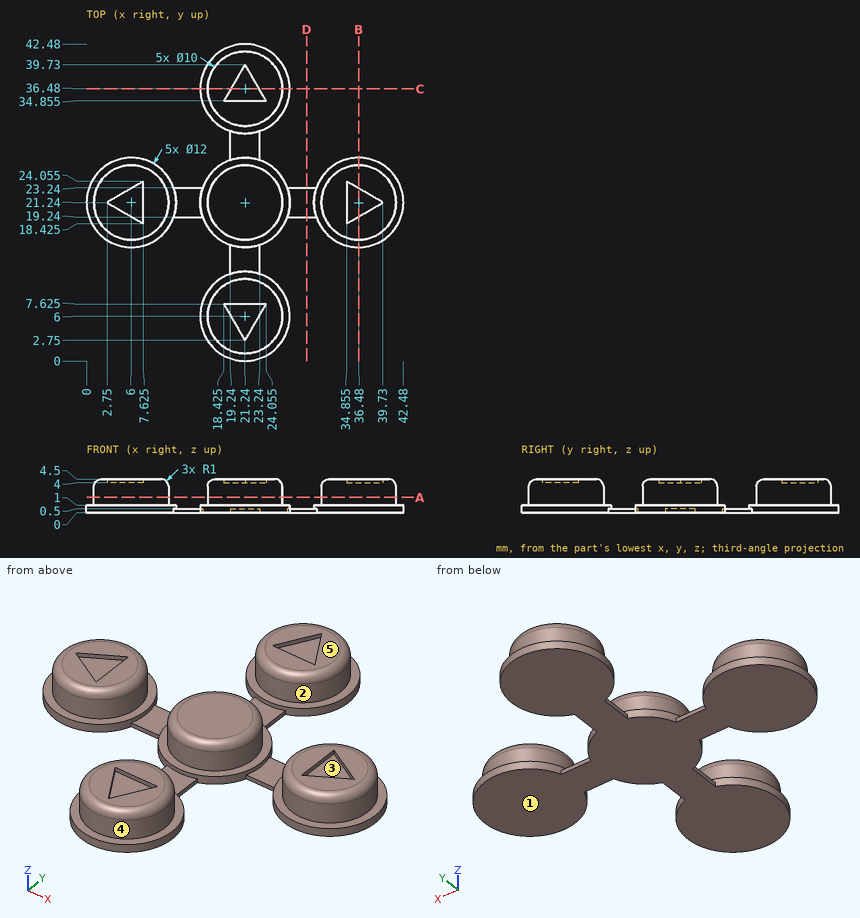
Here's the drawing with two shaded views (mm, measured from the low corner). I have some questions. A direction names the side the tool comes from. Round coordinates to 2 decimals unless told otherwise and drop trailing zeros. Loops run counter-clockwise (first coordinate to the right, second up) from the corner with the lowest first, then second, coordinate; pieces in that order, holes last. Notation, with made-up numbers: M 76,87.25 L 82,87.25 A29 ccw 82,119.25 Z; hole C 43,22 d3. An arc over 180 degrees is marked long. Answer as a JSON object with one key per item and string values. Group by question number.
Q1. Imagine slicing it at A-A, the plane z = 2.05. Please give me the cut outline in (x, y), then the cut area to 3 significant figures.
Q2. We'd pull the mould along X, two halves only. Please class the marked faces 3, 4 and 5: +X half, -X half, draft (parallel to the pull), parting line (faces both ways), or undercut.
Q3. Imagine slicing it at B-B, the plane x = 36.48. Please give me the cut outline in (y, z), then the cut area to 3 significant figures.
Q4. Imagine slicing it at D-D, the plane x = 29.5. Please give me the cut outline in (y, z).
Q5. Will these pins go through, and if not, where does the flat tip stop? pin 1 (5 mm diameter, centred on x = 15.5, y = 10, fed in from +Z); pin 2 (1.5 mm diameter, centred on x = 12, y = 21, fed in from +Z); pin 3 (1.5 mm diameter, centred on y = 36, z = 1, fed in from -X).
Q6. On a 3-axis mill with a long thin cutter (end or side, diameter ignored), from which of +Z, -Z, +X, -X, +Y, -Y can I reach the whole of each face in a straight line? I mean the marked faces 1 and 2. Say none if no direction works.
Q7. Please list where these lines run through material, in increasing order: L1, parallel to X at y = 24.5, z = 0.85; L2, parallel to X at y = 3, z = 1.2; L3, parallel to Z at x = 2.5, y = 25.
Findings:
{
 "1": {"outline": "C 6,21.24 d10; C 21.24,6 d10; C 21.24,21.24 d10; C 21.24,36.48 d10; C 36.48,21.24 d10", "area": "393 mm2"},
 "2": {"face 3": "undercut", "face 4": "parting line", "face 5": "draft"},
 "3": {"outline": "M 15.24,0 L 27.24,0 L 27.24,1 L 26.24,1 L 26.24,3.5 A1 ccw 25.24,4.5 L 23.12,4.5 L 23.12,4 L 19.36,4 L 19.36,4.5 L 17.24,4.5 A1 ccw 16.24,3.5 L 16.24,1 L 15.24,1 Z", "area": "44.7 mm2"},
 "4": {"outline": "M 19.24,0 L 23.24,0 L 23.24,0.5 L 19.24,0.5 Z"},
 "5": {"pin 1": "stops at z = 4.37", "pin 2": "stops at z = 1", "pin 3": "stops at x = 15.24"},
 "6": {"face 1": "-Z, +X, -X, +Y, -Y", "face 2": "+Z"},
 "7": {"L1": "x = 0.96 to 11.04, 16.2 to 26.28, 31.44 to 41.52", "L2": "x = 17.24 to 25.24", "L3": "z = 0 to 1"}
}
